Study the drawing (mm; zero at the part's minimum x, y, z) and answer. A direction names the side the tool comes from. Round coordinates to 2 decimals unless told otherwise and drop trailing zeros. Write each loop counter-clockwise with the first axis right and the second up, starting at its lowest first coordinate (ties: lowest second). Pieces come first, ordered by that corner, then holes.
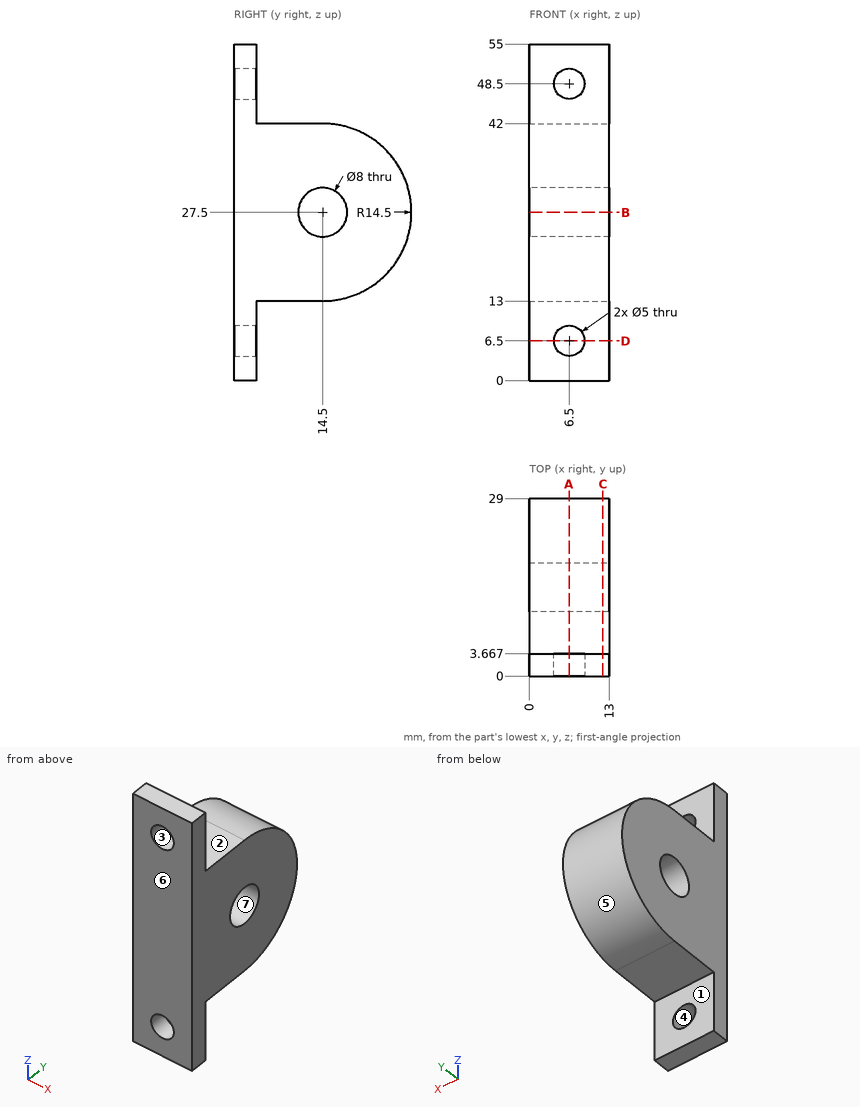
1. For a pull along Z with two mould halves and no side action, classify the marked faces 4, 5, 6 and 7 as released by +Z, released by -Z, zero draft, split by the parting line, or undercut.
Geometry says:
face 4: undercut
face 5: split by the parting line
face 6: zero draft
face 7: undercut
2. Section B-B on z = 27.5 is taken. Determine the outline of the cut face in (x, y), plus the area to 3 significant figures.
Geometry says:
outline: (0, 0) - (13, 0) - (13, 10.5) - (0, 10.5) - close; (0, 18.5) - (13, 18.5) - (13, 29) - (0, 29) - close
area: 273 mm2
3. Section D-D on z = 6.5 is taken. Determine the outline of the cut face in (x, y).
Geometry says:
outline: (0, 0) - (4, 0) - (4, 3.67) - (0, 3.67) - close; (9, 0) - (13, 0) - (13, 3.67) - (9, 3.67) - close
4. Straight lines are drawn through the part: line 1 along Z through (x, y) = (6.5, 1.15); line 2 along X through (y, z) = (2, 48.5); line 3 along Z through (x, y) = (6.5, 14.5). For each, find the intervals that lie inside material, in ascending order.
Geometry says:
line 1: z = 0 to 4, 9 to 46, 51 to 55
line 2: x = 0 to 4, 9 to 13
line 3: z = 13 to 23.5, 31.5 to 42
5. Given pin 1 (1 mm diameter, centred on x = 3.5, z = 19.5, fed in from -Y); pin 2 (4 mm diameter, centred on x = 8.5, y = 18.5, fed in from +Z); pin 3 (6.5 mm diameter, centred on x = 4, z = 50.5, fed in from +Y); pin 4 (6 mm diameter, centred on x = 6, y = 25, fed in from +Z), each flat-ended and moving along its own axis, determine where each tip first touches the part or whether it passes through.
Geometry says:
pin 1: stops at y = 0
pin 2: stops at z = 41.86
pin 3: stops at y = 3.67
pin 4: stops at z = 39.91
6. Section C-C on x = 12 is taken. Determine the outline of the cut face in (y, z).
Geometry says:
outline: (0, 0) - (3.67, 0) - (3.67, 13) - (14.5, 13) arc R14.5 ccw to (14.5, 42) - (3.67, 42) - (3.67, 55) - (0, 55) - close; hole circle Ø8 at (14.5, 27.5)
7. Section A-A on x = 6.5 is taken. Determine the outline of the cut face in (y, z), plus the area to 3 significant figures.
Geometry says:
outline: (0, 0) - (3.67, 0) - (3.67, 4) - (0, 4) - close; (0, 9) - (3.67, 9) - (3.67, 13) - (14.5, 13) arc R14.5 ccw to (14.5, 42) - (3.67, 42) - (3.67, 46) - (0, 46) - close; (0, 51) - (3.67, 51) - (3.67, 55) - (0, 55) - close; hole circle Ø8 at (14.5, 27.5)
area: 759 mm2
8. A tool of negligible diameter and unlimited length cuts with its end or side. For the marked faces 1, 2 and 3, from which of +Z, -Z, +X, -X, +Y, -Y can it reach the whole face along a straight path? Write none if from no direction.
Geometry says:
face 1: -Z, +X, -X, +Y
face 2: +Z, +X, -X, +Y
face 3: +Y, -Y
